Autodesk Inventor part; units mm, degrees
ref_plane "Work Plane1" through (-4.4, 0, 0) normal (1, 0, 0) x (0, 1, 0)
ref_plane "XZ Plane" through (0, 0, 0) normal (0, 1, 0) x (-1, 0, 0)
ref_plane "XY Plane" through (0, 0, 0) normal (0, 0, 1) x (1, 0, 0)
sketch "Sketch1" plane through (0, 0, 0) normal (0, 1, 0) x (-1, 0, 0)
  circle A0 centre (0, 0) radius 2.9
  circle A1 centre (0, -6.1) radius 2.2
  circle A2 centre (0, 6.1) radius 2.2
  circle A3 centre (0, 0) radius 4.4
  circle A4 centre (0, -6.1) radius 3.2
  circle A5 centre (0, 6.1) radius 3.2
  line L0 (-2.5397, -1.4) -> (-3.8533, -2.1241)
  line L1 (-2.5397, 1.4) -> (-3.8533, 2.1241)
  line L2 (1.2, 7.9439) -> (1.7455, 8.782)
  line L3 (-1.2, 7.9439) -> (-1.7455, 8.782)
  point P0 (-2.2223, -3.7975)
  point P1 (2.2223, -3.7975)
  point P2 (2.2223, 3.7975)
  point P3 (-2.2223, 3.7975)
  dimension "d0" = 5.8
  dimension "d1" = 4.4
  dimension "d2" = 4.4
  dimension "d3" = 6.1
  dimension "d4" = 6.1
  dimension "d5" = 1.5
  dimension "d6" = 1
  dimension "d7" = 1
  dimension "d10" = 2.8
  dimension "d11" = 1.4
  dimension "d13" = 2.4
  dimension "d14" = 1.2
extrude "Extrusion1" add sketch "Sketch1" along normal blind 8 contours L1 A3 A5 A0 | A0 A4 A3 L0 | A5 A3 A4 A0 | A5 A3 A2 | A4 A3 A1 | A5 L3 A2 A3 | A3 A2 L2 A5 | A4 A3 A1
fillet "Fillet1" radius 1.5 4 edges at (2.2223, 4, -3.7975) (-2.2223, 4, -3.7975) (-2.2223, 4, 3.7975) (2.2223, 4, 3.7975)
fillet "Fillet2" radius 0.9 1 edges at (3.8533, 4, 2.1241)
fillet "Fillet3" radius 0.5 2 edges at (2.5397, 4, -1.4) (2.5397, 4, 1.4)
fillet "Fillet4" radius 0.7 1 edges at (3.8533, 4, -2.1241)
fillet "Fillet5" radius 0.5 4 edges at (-1.2, 4, 7.9439) (1.2, 4, 7.9439) (-1.7455, 4, 8.782) (1.7455, 4, 8.782)
ref_plane "Work Plane1" through (-4.4, 0, 0) normal (1, 0, 0) x (0, 1, 0)
sketch "Sketch2" plane through (-4.4, 0, 0) normal (1, 0, 0) x (0, 1, 0)
  line L0 (6, -1.0996) -> (6, 0.0004)
  line L1 (6, 0.0004) -> (4, -1.4)
  line L2 (4, -1.4) -> (4, -2.5)
  line L3 (4, -2.5) -> (6, -1.0996)
  line L4 (6, 0.8504) -> (6, 1.9504)
  line L5 (6, 1.9504) -> (2, -0.8504)
  line L6 (2, -0.8504) -> (2, -1.9504)
  line L7 (2, -1.9504) -> (6, 0.8504)
  line L8 (4, 1.4) -> (4, 2.5)
  line L9 (4, 2.5) -> (2, 1.0996)
  line L10 (2, 1.0996) -> (2, -0.0004)
  line L11 (2, -0.0004) -> (4, 1.4)
  line L12 (2, -0.8504) -> (2, -0.0004) construction
  line L13 (6, 0.0004) -> (6, 0.8504) construction
  line L14 (0, -3.0521) -> (0, 3.0521) construction
  point P0 (0, 0)
  point P1 (0, 0)
  point P2 (0, 0)
  dimension "d19" = 125
  dimension "d20" = 4
  dimension "d21" = 5
  dimension "d22" = 0.85
  dimension "d23" = 2.5
  dimension "d24" = 2
extrude "Extrusion2" cut sketch "Sketch2" along normal up to surface
chamfer "Chamfer1" distance 0.5 angle 45 2 edges at (2.2, 8, -6.1) (2.2, 0, -6.1)
chamfer "Chamfer2" distance 0.2 angle 45 40 edges at (-2.9, 8, 0) (2.6007, 8, -1.5722) (3.0635, 8, -1.6887) (3.5317, 8, -2.2372) (3.2777, 8, -2.9354) (2.7696, 8, -3.8497) (0, 8, -9.3) (-2.7696, 8, -3.8497) (-4.4, 8, 0) (-2.7696, 8, 3.8497) (-3.1464, 8, 6.6832) (-1.3695, 8, 7.9935) (0, 8, 3.9) (1.3695, 8, 7.9935) (3.1464, 8, 6.6832) (2.7696, 8, 3.8497) (3.1734, 8, 3.0478) (3.4173, 8, 2.2851) (2.9536, 8, 1.6282) (2.6007, 8, 1.5722) (-3.1464, 0, 6.6832) (-1.3695, 0, 7.9935) (0, 0, 3.9) (1.3695, 0, 7.9935) (3.1464, 0, 6.6832) (2.7696, 0, 3.8497) (3.1734, 0, 3.0478) (3.4173, 0, 2.2851) (2.9536, 0, 1.6282) (2.6007, 0, 1.5722) (-2.9, 0, 0) (2.6007, 0, -1.5722) (3.0635, 0, -1.6887) (3.5317, 0, -2.2372) (3.2777, 0, -2.9354) (2.7696, 0, -3.8497) (0, 0, -9.3) (-2.7696, 0, -3.8497) (-4.4, 0, 0) (-2.7696, 0, 3.8497)
properties part number "umbilicalClip"
Check sheet for the modelled part. Datum: model origin and axes. Units: mm. Coordinates: 2 decimals unless noted, no trailing zeros. Write each loop counter-clockwise with the first axis right and the second up, starting at its lowest first coordinate (ties: lowest second). Pieces come first, ordered by that corner, then holes. Notation, with made-up numbers: (6.5, 72) -> (39.5, 72) arc R15 cw to (39.5, 87) -> close; hole circle Ø1 at (-13.5, 11). An arc over 180 degrees is marked (long way). Use a Markdown table: item, result.
1. Go/stop test with flat-tipped pins: pin 1 Ø1 at (x, y) = (-3, 4.5) entering from +Z; pin 2 Ø1 at (x, z) = (-1.5, -1) entering from -Y; pin 3 Ø1.5 at (y, z) = (7, 5.5) entering from +X; pin 4 Ø2 at (y, z) = (1.5, 1.5) entering from +X. Record where each tip stops, or that it passes through.
Reported:
| item | result |
|---|---|
| pin 1 | stops at z = 8.1 |
| pin 2 | passes through |
| pin 3 | stops at x = 3.2 |
| pin 4 | stops at x = 3.43 |
2. Scan lines: line 1 along Z through (x, y) = (0, 3); line 2 along X through (y, z) = (3, 6.1); line 3 along Z through (x, y) = (1, 1). Record each from-to range of solid material in increasing order.
Reported:
| item | result |
|---|---|
| line 1 | z = -9.3 to -8.3, -3.9 to -2.9, 2.9 to 3.9 |
| line 2 | x = -3.2 to -2.2, 2.2 to 3.2 |
| line 3 | z = -9.14 to -8.06, -4.14 to -2.72, 2.72 to 4.14 |
3. Sectioned sample at D-D (z = -6.1). Enter the section's corners in (x, y), plus the area to 3 significant figures.
Reported:
| item | result |
|---|---|
| outline | (-3.2, 0.2) -> (-3, 0) -> (-2.7, 0) -> (-2.2, 0.5) -> (-2.2, 7.5) -> (-2.7, 8) -> (-3, 8) -> (-3.2, 7.8) -> close; (2.2, 0.5) -> (2.7, 0) -> (3, 0) -> (3.2, 0.2) -> (3.2, 7.8) -> (3, 8) -> (2.7, 8) -> (2.2, 7.5) -> close |
| area | 15.4 mm2 |
4. Sectioned sample at B-B (z = 6.1). Enter the section's corners in (x, y), plus the area to 3 significant figures.
Reported:
| item | result |
|---|---|
| outline | (-3.2, 0.2) -> (-3, 0) -> (-2.4, 0) -> (-2.2, 0.2) -> (-2.2, 7.8) -> (-2.4, 8) -> (-3, 8) -> (-3.2, 7.8) -> close; (2.2, 0.2) -> (2.4, 0) -> (3, 0) -> (3.2, 0.2) -> (3.2, 7.8) -> (3, 8) -> (2.4, 8) -> (2.2, 7.8) -> close |
| area | 15.8 mm2 |
5. Sectioned sample at C-C (y = 5.25). Give the number of separate pieces and of enclosed holes in the cut face, plus the area to 3 significant figures.
Reported:
| item | result |
|---|---|
| separate pieces | 3 |
| enclosed holes | 1 |
| area | 47.7 mm2 |
6. Sectioned sample at A-A (x = 0). Enter the section's corners in (y, z), plus the area to 3 significant figures.
Reported:
| item | result |
|---|---|
| outline | (0, -9.1) -> (0.2, -9.3) -> (7.8, -9.3) -> (8, -9.1) -> (8, -8.8) -> (7.5, -8.3) -> (0.5, -8.3) -> (0, -8.8) -> close; (0, -3.4) -> (0.5, -3.9) -> (7.5, -3.9) -> (8, -3.4) -> (8, -3.1) -> (7.8, -2.9) -> (0.2, -2.9) -> (0, -3.1) -> close; (0, 3.1) -> (0.2, 2.9) -> (7.8, 2.9) -> (8, 3.1) -> (8, 3.7) -> (7.8, 3.9) -> (0.2, 3.9) -> (0, 3.7) -> close |
| area | 23.3 mm2 |
7. Release check for a two-part mould opening along Y. For faces 1 (the flat face through (-2.4, 8, 2.3)), 2 (the flat face through (-3.6, 6, -0.6)), 3 (the cylindrical face through (3.42, 4.05, 2.3)) record: pulls with the +Y half, pulls with the -Y half, needs draft (parallel to the pull), parting line crosses it, or undercut.
Reported:
| item | result |
|---|---|
| face 1 | pulls with the +Y half |
| face 2 | undercut |
| face 3 | needs draft |
